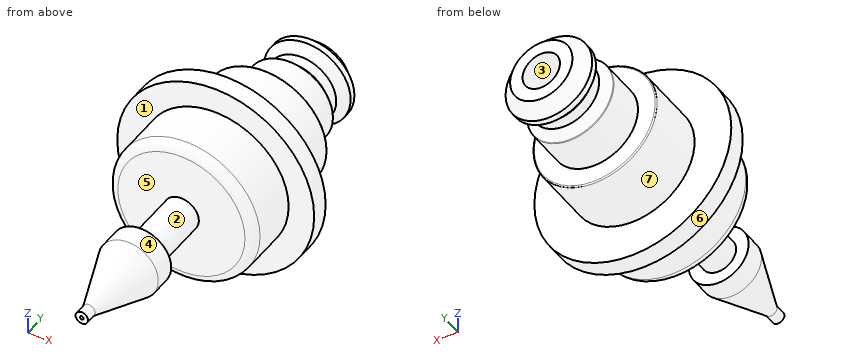
from build123d import *

# Parameters (mm, degrees)
SKETCH_2_R      = 0.5
SKETCH_2_R_2    = 0.15
EXTRUDE_1_DEPTH = 1


with BuildPart() as part:
    # Sketch 1 → Revolve 1 (revolve)
    with BuildSketch(Plane.XY):
        with BuildLine():
            Line((2.4, -9.75), (1.4, -9.75))
            Line((1.4, -9.75), (1.4, -4.5))
            Line((1.4, -4.5), (5.1, -4.5))
            ThreePointArc((5.1, -4.5), (5.630330086, -4.280330086), (5.85, -3.75))
            Line((5.85, -3.75), (5.85, 0))
            Line((5.85, 0), (7.9, 0))
            Line((7.9, 0), (7.9, 1.5))
            Line((7.9, 1.5), (4.955, 1.5))
            Line((4.955, 1.5), (4.955, 6.4))
            ThreePointArc((4.955, 6.4), (4.925710678, 6.470710678), (4.855, 6.5))
            Line((4.855, 6.5), (3.475, 6.5))
            Line((3.475, 6.5), (3.475, 9.65754728))
            ThreePointArc((3.475, 9.65754728), (3.467048751, 9.696624479), (3.444459451, 9.729487426))
            Line((3.444459451, 9.729487426), (2.75, 10.4))
            Line((2.75, 10.4), (2.75, 11.3))
            Line((2.75, 11.3), (3.475, 12))
            Line((3.475, 12), (3.475, 12.5))
            Line((3.475, 12.5), (2.5, 13.5))
            Line((2.5, 13.5), (1.5, 13.5))
            Line((1.5, 13.5), (1.5, 0))
            Line((1.5, 0), (0.15, 0))
            Line((0.15, 0), (0.15, -17.55))
            Line((0.15, -17.55), (2.4, -11.45))
            Line((2.4, -11.45), (2.4, -9.75))
        make_face()
    revolve(axis=Axis((0, 13.5, 0), (0, -1, 0)))

    # Sketch 2 → Extrude 1 (add)
    with BuildSketch(Plane(origin=(0, -17.55, 0), x_dir=(-1, 0, 0), z_dir=(0, -1, 0))):
        with Locations(Location((0, 0, 0), (0, 0, 90))):
            Circle(SKETCH_2_R)
        with Locations(Location((0, 0, 0), (0, 0, 180))):
            Circle(SKETCH_2_R_2, mode=Mode.SUBTRACT)
    extrude(amount=-EXTRUDE_1_DEPTH)


solid = part.part
Part model, mm, in its own coordinate system. Face numbers are marked on the shaded views. A direction names the side the tool comes from. Give positions to 0.01 mm unless a question says otherwise; leave off trailing zeros. Write each loop counter-clockwise with the first axis right and the second up, starting at its lowest first coordinate (ties: lowest second). Pieces come first, ordered by that corner, then holes.
1) Cut at B-B on z = -6.5. Write the cut outline in (x, y), then the cut area to 3 significant figures.
Resolved:
outline: (-4.49, 0) - (4.49, 0) - (4.49, 1.5) - (-4.49, 1.5) - close
area: 13.5 mm2
2) Two-plate mould, pull along Z, no slides. Class the marked faces 1, 2 and 3: released by +Z, released by -Z, zero draft, split by the parting line, or undercut.
Resolved:
face 1: zero draft
face 2: split by the parting line
face 3: undercut
3) Probe L1, parallel to Z at x = 0, y = 10.75; L2, parallel to Z at x = 0, y = 3 (3 decimals); L3, parallel to Y at x = 4.25, z = -0.25. List the from-to ranges inside material, lowest first.
Resolved:
L1: z = -2.75 to -1.5, 1.5 to 2.75
L2: z = -4.955 to -1.5, 1.5 to 4.955
L3: y = -4.5 to 6.5
4) Cut at C-C on y = -9. Write the cut outline in (x, z), then the cut area to 3 significant figures.
Resolved:
outline: circle Ø2.8 at (0, 0); hole circle Ø0.3 at (0, 0)
area: 6.09 mm2
5) Pin check, flat tips, straight feed: pin 1 (1 mm diameter, centred on x = -1, y = 1.5, fed in from -Z); pin 2 (1.4 mm diameter, centred on x = -0.5, z = -0.5, fed in from +Y); pin 3 (1.5 mm diameter, centred on x = -5, z = 3.5, fed in from +Y). Stop position of each tip, or through.
Resolved:
pin 1: stops at z = -7.88
pin 2: stops at y = 0
pin 3: stops at y = 1.5
6) Which spindle directions (+Z, -Z, +X, -X, +Y, -Y) get a long thin tool onto all of the face, cutting with end or side? Do the marked faces 4, 5, 6 and 7. Say none if no direction does.
Resolved:
face 4: -Y
face 5: none
face 6: +Y, -Y
face 7: +Y
7) Cut at A-A on y = 0.5. Write the cut outline in (x, z), then the cut area to 3 significant figures.
Resolved:
outline: circle Ø15.8 at (0, 0); hole circle Ø3 at (0, 0)
area: 189 mm2
